from build123d import *

# Parameters (mm, degrees)
F1_DEPTH = 7.112


with BuildPart() as f1:
    # F0 (on Top) → F1 (new body)
    with BuildSketch(Plane.XY):
        with BuildLine():
            Line((-55.80807, -4.691954), (54.014004, -4.691954))
            ThreePointArc((54.014004, -4.691954), (77.989111, -0.015025), (54.025366, 4.719774))
            Line((54.025366, 4.719774), (-55.818372, 4.719774))
            ThreePointArc((-55.818372, 4.719774), (-70.124067, 13.45667), (-81.978054, 1.604697))
            Line((-81.978054, 1.604697), (-75.612001, 4.942868))
            Line((-75.612001, 4.942868), (-67.786179, 8.611853))
            Line((-67.786179, 8.611853), (-60.695834, 3.668985))
            Line((-60.695834, 3.668985), (-61.431311, -4.942868))
            Line((-61.431311, -4.942868), (-69.257133, -8.611853))
            Line((-69.257133, -8.611853), (-75.452484, -11.645313))
            ThreePointArc((-75.452484, -11.645313), (-63.999779, -12.775067), (-55.80807, -4.691954))
        make_face()
        Polygon((55.007732, 0), (60.275092, 9.123336), (70.809812, 9.123336), (76.077173, 0), (70.809812, -9.123336), (60.275092, -9.123336), align=None, mode=Mode.SUBTRACT)
    extrude(amount=F1_DEPTH)


solid = f1.part
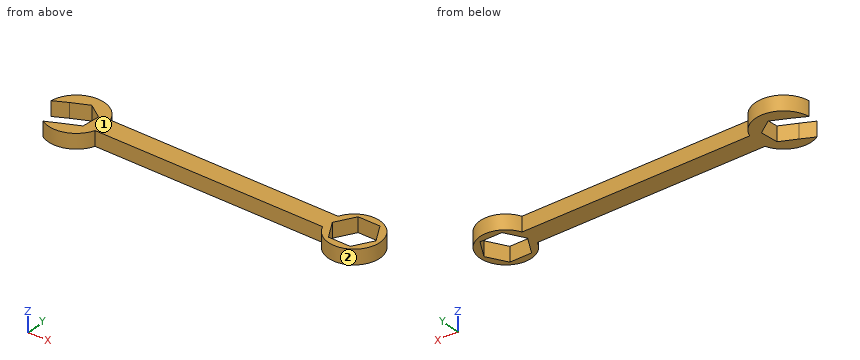
Work out the finished part from the listing and answer in its coordinate system (mm). Face numbers are marked on the shaded views. Give positions to 0.01 mm unless a question says otherwise; leave off trailing zeros. Loops run counter-clockwise (first coordinate to the right, second up) from the corner with the lowest first, then second, coordinate; pieces in that order, holes last. Notation, with made-up numbers: (36, -20.75) - (91, -20.75) arc R25 ccw to (91, 0.25) - close; hole circle Ø7 at (2.25, -4.5). An arc over 180 degrees is marked (long way). Answer in a Markdown table with one row per item. Add a question column.
Q1. Each of these flat-tipped pins is pushed along its axis until it touches: P1, Ø2, axis at x = -7.5, z = 4, coming from the +Y side; P2, Ø3, axis at y = -0.5, z = 2, coming from the -X side; P3, Ø3.5, axis at x = 10, z = 4.5, coming from the -Y side. Where does it stop, or does it pass through?
Q2. The part is cut by section C-C (y = 10.5). Determine the outline of the cut face in (x, z), and give its area (3 significant figures).
Q3. Determine the mould class of the marked faces 1 and 2 for opening direction X: released by +X, released by -X, zero draft, split by the parting line, or undercut.
Q4. The part is cut by section B-B (x = 66). Determine the outline of the cut face in (y, z), and give its area (3 significant figures).
Q5. The part is cut by section A-A (z = 2). Determine the outline of the cut face in (x, y).
Q6. Consider line 1 along X through (y, z) = (-9, 6.75); line 2 along X through (y, z) = (-7.75, 2.5); line 3 along Y through (x, z) = (-42, 0.75). Determine where each line is inside the solid, lowest interval first.
Q7. The part is cut by section D-D (x = -31.5). Determine the outline of the cut face in (y, z), and give its area (3 significant figures).
Solution:
| question | item | result |
|---|---|---|
| 1 | P1 | stops at y = 4.72 |
| 1 | P2 | stops at x = -61.18 |
| 1 | P3 | stops at y = -4.69 |
| 2 | outline | (-77.09, 0) - (-59.95, 0) - (-59.95, 7.11) - (-77.09, 7.11) - close; (58.86, 0) - (72.23, 0) - (72.23, 7.11) - (58.86, 7.11) - close |
| 2 | area | 217 mm² |
| 3 | face 1 | zero draft |
| 3 | face 2 | undercut |
| 4 | outline | (-12.44, 0) - (-9.12, 0) - (-9.12, 7.11) - (-12.44, 7.11) - close; (9.12, 0) - (12.44, 0) - (12.44, 7.11) - (9.12, 7.11) - close |
| 4 | area | 47.2 mm² |
| 5 | outline | (-81.98, 1.6) - (-75.61, 4.94) - (-67.79, 8.61) - (-60.7, 3.67) - (-61.43, -4.94) - (-69.26, -8.61) - (-75.45, -11.65) arc R13.55 ccw to (-55.81, -4.69) - (54.01, -4.69) arc R12.45 ccw (long way) to (54.03, 4.72) - (-55.82, 4.72) arc R13.55 ccw to start; hole (55.01, 0) - (60.28, -9.12) - (70.81, -9.12) - (76.08, 0) - (70.81, 9.12) - (60.28, 9.12) - close |
| 6 | line 1 | x = -70.05 to -58.39, 56.94 to 60.2, 70.88 to 74.14 |
| 6 | line 2 | x = -67.42 to -57.4, 55.8 to 59.48, 71.6 to 75.28 |
| 6 | line 3 | y = -4.69 to 4.72 |
| 7 | outline | (-4.69, 0) - (4.72, 0) - (4.72, 7.11) - (-4.69, 7.11) - close |
| 7 | area | 66.9 mm² |
